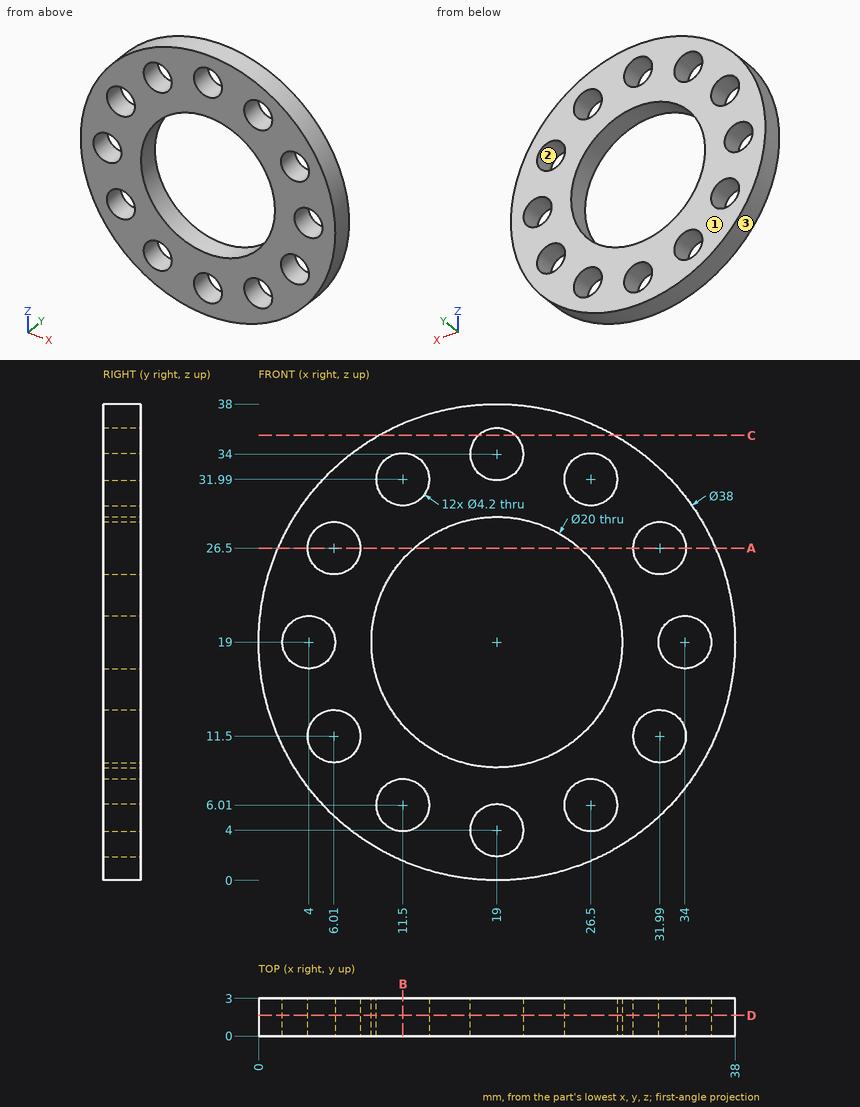
Design review of the part shown in the three views and the two pictorial views. Dimensions are in mm from the part's minimum x, y and z. Round coordinates to 2 decimals unless told otherwise and drop trailing zeros. Loops run counter-clockwise (first coordinate to the right, second up) from the corner with the lowest first, then second, coordinate; pieces in that order, holes last.
Q1. Add section D-D on y = 1.65. Give the number of separate pieces and of enclosed holes in the cut face.
Result sheet:
separate pieces: 1
enclosed holes: 13
Q2. Mouldability with a two-part tool opening along Z and no side actions: class the marked faces 1, 2 and 3 as +Z half, -Z half, draft (parallel to the pull), parting line (faces both ways), or undercut.
Result sheet:
face 1: draft
face 2: undercut
face 3: parting line
Q3. To check wall thickness, follow line 1 along X through (y, z) = (1.5, 19); line 2 along X through (y, z) = (1, 26.5) (1 decimal). State the ranges of each line that lie inside material, in increasing order.
Result sheet:
line 1: x = 0 to 1.9, 6.1 to 9, 29 to 31.9, 36.1 to 38
line 2: x = 1.5 to 3.9, 8.1 to 12.4, 25.6 to 29.9, 34.1 to 36.5
Q4. Insertion check: pin 1 Ø1.5 at (y, z) = (1.5, 15.5) entering from +X. The pin has a flat end and moves straight along its axis. Give the tip position at first contact, or say it passes through.
Result sheet:
pin 1: stops at x = 37.8
Q5. Add section C-C on z = 35.5. Write out the cut boundary in (x, y).
Result sheet:
outline: (9.58, 0) - (17.53, 0) - (17.53, 3) - (9.58, 3) - close; (20.47, 0) - (28.42, 0) - (28.42, 3) - (20.47, 3) - close
Q6. Add section A-A on z = 26.5. Write out the cut boundary in (x, y) (1 decimal).
Result sheet:
outline: (1.5, 0) - (3.9, 0) - (3.9, 3) - (1.5, 3) - close; (8.1, 0) - (12.4, 0) - (12.4, 3) - (8.1, 3) - close; (25.6, 0) - (29.9, 0) - (29.9, 3) - (25.6, 3) - close; (34.1, 0) - (36.5, 0) - (36.5, 3) - (34.1, 3) - close
Q7. Add section B-B on x = 11.5. Write out the cut boundary in (y, z) (1 decimal).
Result sheet:
outline: (0, 1.5) - (3, 1.5) - (3, 3.9) - (0, 3.9) - close; (0, 8.1) - (3, 8.1) - (3, 12.4) - (0, 12.4) - close; (0, 25.6) - (3, 25.6) - (3, 29.9) - (0, 29.9) - close; (0, 34.1) - (3, 34.1) - (3, 36.5) - (0, 36.5) - close
